Autodesk Inventor part; units mm, degrees
ref_plane "YZ Plane" through (0, 0, 0) normal (1, 0, 0) x (0, 1, 0)
ref_plane "XZ Plane" through (0, 0, 0) normal (0, 1, 0) x (-1, 0, 0)
ref_plane "XY Plane" through (0, 0, 0) normal (0, 0, 1) x (1, 0, 0)
sketch "Sketch1" plane through (0, 0, 0) normal (0, 0, 1) x (1, 0, 0)
  circle A0 centre (0, 0) radius 12.5
  circle A1 centre (-30, 0) radius 3
  circle A2 centre (-15, -25.9808) radius 3
  circle A3 centre (15, -25.9808) radius 3
  circle A4 centre (30, 0) radius 3
  circle A5 centre (15, 25.9808) radius 3
  circle A6 centre (-15, 25.9808) radius 3
  line L0 (0, 57.5) -> (49.7965, 28.75)
  line L1 (49.7965, 28.75) -> (49.7965, -28.75)
  line L2 (49.7965, -28.75) -> (0, -57.5)
  line L3 (0, -57.5) -> (-49.7965, -28.75)
  line L4 (-49.7965, -28.75) -> (-49.7965, 28.75)
  line L5 (-49.7965, 28.75) -> (0, 57.5)
  point P0 (49.7965, 0)
  dimension "d0" = 25
  dimension "d2" = 6
  dimension "d6" = 360
  dimension "d15" = 30
  dimension "d33" = 115
extrude "Extrusion1" add sketch "Sketch1" along normal blind 10 contours A1 | A2 | A3 | A4 | A5 | A6 | L0 L1 L2 L3 L4 L5
sketch "Sketch7" plane through (0, 0, 10) normal (0, 0, 1) x (1, 0, 0)
  circle A0 centre (0, 51) radius 3
  circle A1 centre (-44.1673, 25.5) radius 3
  circle A2 centre (-44.1673, -25.5) radius 3
  circle A3 centre (0, -51) radius 3
  circle A4 centre (44.1673, -25.5) radius 3
  circle A5 centre (44.1673, 25.5) radius 3
  line L0 (0, 51) -> (0, -51)
  point P0 (0, 0)
  dimension "d42" = 6
  dimension "d46" = 360
  dimension "d96" = 102
extrude "Extrusion6" cut sketch "Sketch7" against normal through all
sketch "Sketch9" plane through (0, 0, 0) normal (0, 0, -1) x (-1, 0, 0)
  circle A0 centre (0, 0) radius 25
  dimension "d56" = 50
extrude "Extrusion8" cut sketch "Sketch9" against normal blind 5
sketch "Sketch14" plane through (0, 0, 10) normal (0, 0, 1) x (1, 0, 0)
  circle A0 centre (-45.7965, 0) radius 2.5
  circle A1 centre (-22.8982, -39.6609) radius 2.5
  circle A2 centre (22.8982, -39.6609) radius 2.5
  circle A3 centre (45.7965, 0) radius 2.5
  circle A4 centre (22.8982, 39.6609) radius 2.5
  circle A5 centre (-22.8982, 39.6609) radius 2.5
  line L0 (-49.7965, 28.75) -> (-49.7965, -28.75)
  point P0 (0, 0)
  point P1 (-45.7965, 0)
  dimension "d81" = 5
  dimension "d85" = 360
  dimension "d97" = 4
extrude "Extrusion13" cut sketch "Sketch14" against normal through all
sketch "Sketch15" plane through (0, 0, 10) normal (0, 0, 1) x (1, 0, 0)
  circle A0 centre (-22.8982, 39.6609) radius 2.5
  circle A1 centre (-22.8982, 39.6609) radius 6.5
  circle A2 centre (-45.7965, 0) radius 6.5
  circle A3 centre (-22.8982, -39.6609) radius 6.5
  circle A4 centre (22.8982, -39.6609) radius 6.5
  circle A5 centre (45.7965, 0) radius 6.5
  circle A6 centre (22.8982, 39.6609) radius 6.5
  point P0 (0, 0)
  dimension "d89" = 13
  dimension "d92" = 360
extrude "Extrusion14" cut sketch "Sketch15" against normal blind 5 contours A0 | A1 | A2 | A3 | A4 | A5 | A6
sketch "Sketch16" plane through (0, 0, 5) normal (0, 0, 1) x (1, 0, 0)
  line L0 (-29.3353, 40.5633) -> (-20.4612, 45.6867)
  arc A0 (-29.3353, 40.5633) -> (-20.4612, 45.6867) centre (-22.8982, 39.6609) ccw
  circle A1 centre (-22.8982, 39.6609) radius 2.5
  line L1 (49.7965, 5.1235) -> (49.7965, -5.1235)
  arc A2 (49.7965, 5.1235) -> (49.7965, -5.1235) centre (45.7965, 0) ccw
  circle A3 centre (45.7965, 0) radius 2.5
  line L2 (-20.4612, -45.6867) -> (-29.3353, -40.5633)
  arc A4 (-20.4612, -45.6867) -> (-29.3353, -40.5633) centre (-22.8982, -39.6609) ccw
  circle A5 centre (-22.8982, -39.6609) radius 2.5
  point P0 (0, 0)
extrude "Extrusion15" add sketch "Sketch16" along normal blind 5
sketch "Sketch17" plane through (0, 0, 10) normal (0, 0, 1) x (1, 0, 0)
  circle A0 centre (-22.8982, 39.6609) radius 2.5
  circle A1 centre (45.7965, 0) radius 2.5
  circle A2 centre (-22.8982, -39.6609) radius 2.5
  point P0 (0, 0)
extrude "Extrusion16" add sketch "Sketch17" against normal blind 10
sketch "Sketch18" plane through (0, 0, 5) normal (0, 0, -1) x (-1, 0, 0)
  circle A0 centre (0, 0) radius 12.5
  circle A1 centre (0, 0) radius 25
extrude "Extrusion17" add sketch "Sketch18" along normal blind 5
sketch "Sketch19" plane through (0, 0, 5) normal (0, 0, 1) x (1, 0, 0)
  line L0 (-49.7965, -5.1235) -> (-49.7965, 5.1235)
  arc A0 (-49.7965, -5.1235) -> (-49.7965, 5.1235) centre (-45.7965, 0) ccw
  circle A1 centre (-45.7965, 0) radius 2.5
  line L1 (20.4612, 45.6867) -> (29.3353, 40.5633)
  arc A2 (20.4612, 45.6867) -> (29.3353, 40.5633) centre (22.8982, 39.6609) ccw
  circle A3 centre (22.8982, 39.6609) radius 2.5
  line L2 (29.3353, -40.5633) -> (20.4612, -45.6867)
  arc A4 (29.3353, -40.5633) -> (20.4612, -45.6867) centre (22.8982, -39.6609) ccw
  circle A5 centre (22.8982, -39.6609) radius 2.5
  point P0 (0, 0)
extrude "Extrusion18" add sketch "Sketch19" along normal blind 5 contours L0 A0 | A1 | L1 A2 | A3 | L2 A4 | A5
sketch "Sketch20" plane through (22.8982, 39.6609, 5) normal (0, 0, -1) x (-1, 0, 0)
  circle A0 centre (0, 0) radius 2.5
  circle A1 centre (0, -79.3218) radius 2.5
  circle A2 centre (68.6947, -39.6609) radius 2.5
  point P0 (22.8982, -39.6609)
extrude "Extrusion19" add sketch "Sketch20" along normal blind 5
sketch "Sketch24" plane through (0, 0, 0) normal (0, 0, -1) x (-1, 0, 0)
  circle A0 centre (-22.8982, -39.6609) radius 2.5
  line L0 (-22.8982, -39.6609) -> (-24.8982, -43.125) construction
  line L1 (-49.7965, -28.75) -> (0, -57.5)
  circle A1 centre (22.8982, -39.6609) radius 2.5
  line L2 (22.8982, -39.6609) -> (24.8982, -43.125) construction
  circle A2 centre (45.7965, 0) radius 2.5
  line L3 (45.7965, 0) -> (49.7965, 0) construction
  circle A3 centre (22.8982, 39.6609) radius 2.5
  line L4 (22.8982, 39.6609) -> (24.8982, 43.125) construction
  circle A4 centre (-22.8982, 39.6609) radius 2.5
  line L5 (-22.8982, 39.6609) -> (-24.8982, 43.125) construction
  circle A5 centre (-45.7965, 0) radius 2.5
  line L6 (-45.7965, 0) -> (-49.7965, 0) construction
  point P0 (0, 0)
  dimension "d130" = 5
  dimension "d131" = 4
  dimension "d134" = 360
extrude "Extrusion22" cut sketch "Sketch24" against normal through all contours A0 | A2 | A4
sketch "Sketch26" plane through (0, 0, 10) normal (0, 0, 1) x (1, 0, 0)
  circle A0 centre (-45.7965, 0) radius 2.5
  circle A1 centre (-45.7965, 0) radius 7.5
  circle A2 centre (22.8982, -39.6609) radius 7.5
  circle A3 centre (22.8982, 39.6609) radius 7.5
  point P0 (0, 0)
  dimension "d141" = 15
  dimension "d147" = 360
extrude "Extrusion23" cut sketch "Sketch26" against normal blind 5 contours A0 | A1 | A2 | A3
properties part number "TA01" material "ABS Plastic"
The listing builds one solid part. Answer for the finished solid, in the listing's coordinates (mm). A direction names the side the tool comes from. Round coordinates to 2 decimals unless told otherwise and drop trailing zeros. Write each loop counter-clockwise with the first axis right and the second up, starting at its lowest first coordinate (ties: lowest second). Pieces come first, ordered by that corner, then holes. Notation, with made-up numbers: (30, -18) - (62, -18) arc R26 ccw to (62, 18) - close; hole circle Ø8 at (-28.5, -37.5). An arc over 180 degrees is marked (long way). Use a Markdown table: item, result. Add a question column.
1. For a pull along X with two mould halves and no side action, classify faces 3 (the face through (-49.796, 0, 4)), 4 (the face through (49.796, 0, 5)), 5 (the face through (41.17, -25.37, 5.07)), 6 (the face through (10, -12, 10)) as +X half, -X half, draft (parallel to the pull), parting line (faces both ways), or undercut.
2. Flat-ended cylindrical pins translate along their axes: P1, Ø3, axis at x = 1, z = 5.5, coming from the +Y side; P2, Ø13.5, axis at x = 22.9, y = -39.66, coming from the +Z side; P3, Ø3, axis at y = -31, z = 7.5, coming from the +X side. Find the tip coordinate at first contact, or state that the pin passes through.
3. The part is cut by section A-A (y = 51). Write down the section's boundary in (x, z), and give its area (3 significant figures).
4. A tool of negligible diameter and unlimited length cuts with its end or side. For faces 1 (the face through (21.1, -37.6, 5)), 2 (the face through (-43.3, 0.1, 2.5)), from which of +Z, -Z, +X, -X, +Y, -Y can it reach the whole face along a straight path? Write none if from no direction.
5. The part is cut by section C-C (x = 1.5). Write down the section's boundary in (y, z).
6. The part is cut by section B-B (z = 8). Write down the section's boundary in (x, y).
7. The part is cut by section D-D (y = -44). Write down the section's boundary in (x, z).
8. Consider line 1 (Y direction, x = 0, z = 5.5); line 2 (Y direction, x = 46, z = 9.75); line 3 (X direction, y = -27, z = 7.75). Determine where each line is inside the solid, lowest interval first.
Reported:
| question | item | result |
|---|---|---|
| 1 | face 3 | -X half |
| 1 | face 4 | +X half |
| 1 | face 5 | undercut |
| 1 | face 6 | draft |
| 2 | P1 | y = 57.5 |
| 2 | P2 | z = 5 |
| 2 | P3 | x = 48.5 |
| 3 | outline | (-11.26, 0) - (-3, 0) - (-3, 10) - (-11.26, 10) - close; (3, 0) - (11.26, 0) - (11.26, 10) - (3, 10) - close |
| 3 | area | 165 mm^2 |
| 4 | face 1 | +Z |
| 4 | face 2 | +Z, -Z |
| 5 | outline | (-56.63, 0) - (-53.6, 0) - (-53.6, 10) - (-56.63, 10) - close; (-48.4, 0) - (-12.41, 0) - (-12.41, 10) - (-48.4, 10) - close; (12.41, 0) - (48.4, 0) - (48.4, 10) - (12.41, 10) - close; (53.6, 0) - (56.63, 0) - (56.63, 10) - (53.6, 10) - close |
| 6 | outline | (-49.8, -28.75) - (-29.34, -40.56) - (-20.46, -45.69) - (0, -57.5) - (19.4, -46.3) arc R7.5 cw (long way) to (30.39, -39.95) - (49.8, -28.75) - (49.8, 28.75) - (30.39, 39.95) arc R7.5 cw (long way) to (19.4, 46.3) - (0, 57.5) - (-20.46, 45.69) - (-29.34, 40.56) - (-49.8, 28.75) - (-49.8, 6.34) arc R7.5 cw (long way) to (-49.8, -6.34) - close; hole circle Ø6 at (-44.17, -25.5); hole circle Ø6 at (-44.17, 25.5); hole circle Ø25 at (0, 0); hole circle Ø6 at (0, -51); hole circle Ø6 at (0, 51); hole circle Ø6 at (44.17, -25.5); hole circle Ø6 at (44.17, 25.5) |
| 7 | outline | (-23.38, 0) - (23.38, 0) - (23.38, 5) - (16.78, 5) - (16.78, 10) - (-23.38, 10) - close |
| 8 | line 1 | -57.5 to -54, -48 to -12.5, 12.5 to 48, 54 to 57.5 |
| 8 | line 2 | -30.94 to -27.88, -23.12 to 23.12, 27.88 to 30.94 |
| 8 | line 3 | -49.8 to -46.77, -41.57 to 41.57, 46.77 to 49.8 |
